from build123d import *

# Parameters (mm, degrees)
SKETCH_1_W          = 120
SKETCH_1_H          = 60
EXTRUDE_1_DEPTH     = 2.5
SKETCH_1_3_W        = 120
SKETCH_1_3_H        = 60
EXTRUDE_2_DEPTH     = 27.5
SKETCH_2_R          = 1.7
CUT_EXTRUDE_1_DEPTH = 74.484692283
SKETCH_3_R          = 1.7
CUT_EXTRUDE_2_DEPTH = 73.5
CUT_EXTRUDE_3_DEPTH = 0.5
SKETCH_5_W          = 2.5
SKETCH_5_H          = 12
CUT_EXTRUDE_4_DEPTH = 8.5
SKETCH_6_R          = 3
CUT_EXTRUDE_5_DEPTH = 15
CHAMFER_1_SIZE      = 2


with BuildPart() as part:
    # 草图1 → 凸台-拉伸1 (new body)
    with BuildSketch(Plane.XY):
        Rectangle(SKETCH_1_W, SKETCH_1_H)
    extrude(amount=-EXTRUDE_1_DEPTH)

    # 草图1<3> → 凸台-拉伸2 (add)
    with BuildSketch(Plane.XY):
        Rectangle(SKETCH_1_3_W, SKETCH_1_3_H)
        with BuildLine():
            Line((-52, 27.5), (52, 27.5))
            Line((52, 27.5), (52, 26))
            ThreePointArc((52, 26), (53.171572875, 23.171572875), (56, 22))
            Line((56, 22), (57.5, 22))
            Line((57.5, 22), (57.5, -22))
            Line((57.5, -22), (56, -22))
            ThreePointArc((56, -22), (53.171572875, -23.171572875), (52, -26))
            Line((52, -26), (52, -27.5))
            Line((52, -27.5), (-52, -27.5))
            Line((-52, -27.5), (-52, -26))
            ThreePointArc((-52, -26), (-53.171572875, -23.171572875), (-56, -22))
            Line((-56, -22), (-57.5, -22))
            Line((-57.5, -22), (-57.5, 22))
            Line((-57.5, 22), (-56, 22))
            ThreePointArc((-56, 22), (-53.171572875, 23.171572875), (-52, 26))
            Line((-52, 26), (-52, 27.5))
        make_face(mode=Mode.SUBTRACT)
    extrude(amount=EXTRUDE_2_DEPTH)

    # 草图2 → 切除-拉伸1 (cut, through all)
    with BuildSketch(Plane.XY.offset(27.5)):
        with Locations((-56, 26)):
            Circle(SKETCH_2_R)
        with Locations((56, 26)):
            Circle(SKETCH_2_R)
        with Locations((56, -26)):
            Circle(SKETCH_2_R)
        with Locations((-56, -26)):
            Circle(SKETCH_2_R)
    extrude(amount=-CUT_EXTRUDE_1_DEPTH, mode=Mode.SUBTRACT)

    # 草图3 → 切除-拉伸2 (cut, through all)
    with BuildSketch(Plane.XY):
        with Locations((-5, 7.5)):
            Circle(SKETCH_3_R)
        with BuildLine():
            Line((52.5, 9.2), (53.5, 9.2))
            ThreePointArc((53.5, 9.2), (55.2, 7.5), (53.5, 5.8))
            Line((53.5, 5.8), (52.5, 5.8))
            ThreePointArc((52.5, 5.8), (50.8, 7.5), (52.5, 9.2))
        make_face()
        with BuildLine():
            Line((52.5, -5.8), (53.5, -5.8))
            ThreePointArc((53.5, -5.8), (55.2, -7.5), (53.5, -9.2))
            Line((53.5, -9.2), (52.5, -9.2))
            ThreePointArc((52.5, -9.2), (50.8, -7.5), (52.5, -5.8))
        make_face()
    extrude(amount=-CUT_EXTRUDE_2_DEPTH, mode=Mode.SUBTRACT)

    # 草图4 → 切除-拉伸3 (cut)
    with BuildSketch(Plane.XY):
        Polygon((-1.8, 7.5), (-3.4, 10.271281292), (-6.6, 10.271281292), (-8.2, 7.5), (-6.6, 4.728718708), (-3.4, 4.728718708), align=None)
        Polygon((56.2, 7.5), (54.6, 10.271281292), (51.4, 10.271281292), (49.8, 7.5), (51.4, 4.728718708), (54.6, 4.728718708), align=None)
        Polygon((56.2, -7.5), (54.6, -4.728718708), (51.4, -4.728718708), (49.8, -7.5), (51.4, -10.271281292), (54.6, -10.271281292), align=None)
    extrude(amount=-CUT_EXTRUDE_3_DEPTH, mode=Mode.SUBTRACT)

    # 草图5 → 切除-拉伸4 (cut)
    with BuildSketch(Plane.XY.offset(27.5)):
        with Locations((58.75, 0)):
            Rectangle(SKETCH_5_W, SKETCH_5_H)
    extrude(amount=-CUT_EXTRUDE_4_DEPTH, mode=Mode.SUBTRACT)

    # 草图6 → 切除-拉伸5 (cut)
    with BuildSketch(Plane(origin=(0, 0, -2.5), x_dir=(-1, 0, 0), z_dir=(0, 0, -1))):
        with Locations((-56, 26)):
            Circle(SKETCH_6_R)
        with Locations((-56, -26)):
            Circle(SKETCH_6_R)
        with Locations((56, -26)):
            Circle(SKETCH_6_R)
        with Locations((56, 26)):
            Circle(SKETCH_6_R)
    extrude(amount=-CUT_EXTRUDE_5_DEPTH, mode=Mode.SUBTRACT)

    # 倒角1
    # the kernel refuses this chamfer: 2 mm, written as the material it takes off along each edge
    with BuildSketch(Plane(origin=(-56, 26, 12.5), x_dir=(1, 0, 0), z_dir=(0, -1, 0))) as chamfer_1_piece_1_section:
        Polygon((1.7, CHAMFER_1_SIZE), (1.7 + CHAMFER_1_SIZE, 0), (1.7, 0), align=None)
    chamfer_1_piece_1 = revolve(axis=Axis((-56, 26, 12.5), (0, 0, 1)), mode=Mode.PRIVATE)
    chamfer_1_piece_1 = chamfer_1_piece_1 & Plane(origin=(-56, 26, 13.857190975), x_dir=(-1, 0, 0), z_dir=(0, 0, -1)) * Cylinder(3, 15, mode=Mode.PRIVATE)
    add(chamfer_1_piece_1, mode=Mode.SUBTRACT)
    with BuildSketch(Plane(origin=(-56, -26, 12.5), x_dir=(1, 0, 0), z_dir=(0, -1, 0))) as chamfer_1_piece_2_section:
        Polygon((1.7, CHAMFER_1_SIZE), (1.7 + CHAMFER_1_SIZE, 0), (1.7, 0), align=None)
    chamfer_1_piece_2 = revolve(axis=Axis((-56, -26, 12.5), (0, 0, 1)), mode=Mode.PRIVATE)
    chamfer_1_piece_2 = chamfer_1_piece_2 & Plane(origin=(-56, -26, 13.857190975), x_dir=(-1, 0, 0), z_dir=(0, 0, -1)) * Cylinder(3, 15, mode=Mode.PRIVATE)
    add(chamfer_1_piece_2, mode=Mode.SUBTRACT)
    with BuildSketch(Plane(origin=(56, -26, 12.5), x_dir=(1, 0, 0), z_dir=(0, -1, 0))) as chamfer_1_piece_3_section:
        Polygon((1.7, CHAMFER_1_SIZE), (1.7 + CHAMFER_1_SIZE, 0), (1.7, 0), align=None)
    chamfer_1_piece_3 = revolve(axis=Axis((56, -26, 12.5), (0, 0, 1)), mode=Mode.PRIVATE)
    chamfer_1_piece_3 = chamfer_1_piece_3 & Plane(origin=(56, -26, 13.857190975), x_dir=(-1, 0, 0), z_dir=(0, 0, -1)) * Cylinder(3, 15, mode=Mode.PRIVATE)
    add(chamfer_1_piece_3, mode=Mode.SUBTRACT)
    with BuildSketch(Plane(origin=(56, 26, 12.5), x_dir=(1, 0, 0), z_dir=(0, -1, 0))) as chamfer_1_piece_4_section:
        Polygon((1.7, CHAMFER_1_SIZE), (1.7 + CHAMFER_1_SIZE, 0), (1.7, 0), align=None)
    chamfer_1_piece_4 = revolve(axis=Axis((56, 26, 12.5), (0, 0, 1)), mode=Mode.PRIVATE)
    chamfer_1_piece_4 = chamfer_1_piece_4 & Plane(origin=(56, 26, 13.857190975), x_dir=(-1, 0, 0), z_dir=(0, 0, -1)) * Cylinder(3, 15, mode=Mode.PRIVATE)
    add(chamfer_1_piece_4, mode=Mode.SUBTRACT)


solid = part.part
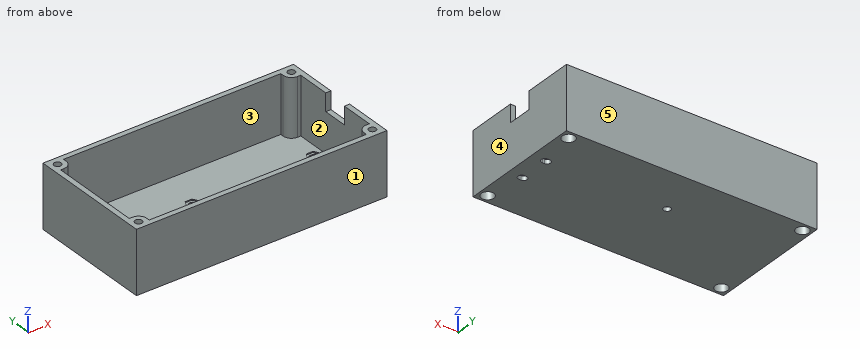
Design review of the part built by this model. Coordinates are the model's own, in mm. Face numbers are marked on the shaded views. A direction names the side the tool comes from. Give positions to 0.01 mm unless a question says otherwise; leave off trailing zeros. Write each loop counter-clockwise with the first axis right and the second up, starting at its lowest first coordinate (ties: lowest second). Pieces come first, ordered by that corner, then holes. Notation, with made-up numbers: M 87.25,20.25 L 129.25,20.25 A20 cw 129.25,45.25 Z; hole C 60.5,72 d10. An arc over 180 degrees is marked long. Answer as a JSON object with one key per item and string values. Group by question number.
1) Clearance check with flat-ended pins moving along their axes: pin 1 Ø3.5 at (x, y) = (56, -26) entering from -Z; pin 2 Ø6 at (x, y) = (-30, -18) entering from +Z. State where each tip first meets the part, or that it passes through.
2) We need section B-B (z = 3). Give the boundary of the cut face in (x, y), and give its area (3 significant figures).
3) We need section C-C (y = -3.5). Give the boundary of the cut face in (x, z), and give its area (3 significant figures).
4) We need section A-A (x = -5). Give the boundary of the cut face in (y, z).
5) We need section D-D (x = -47.5). Give the boundary of the cut face in (y, z).
6) Mouldability with a two-part tool opening along Y and no side actions: class the marked faces 3, 4 and 5 as released by +Y, released by -Y, zero draft, split by the parting line, or undercut.
7) For line 1 along Y through (x, z) = (-56, 20.25); line 2 along X through (y, z) = (26, 8.75); line 3 along Y through (x, z) = (56, 0.75), list the stretches that pass through material, from the lowest coordinate up.
8) Tool access review of the marked faces 1 and 2: name each direction out of +Z, -Z, +X, -X, +Y, -Y from which nothing blocks a thin tool from reaching the whole face with its end or side.
Answer key:
{
 "1": {"pin 1": "stops at z = 14.45", "pin 2": "stops at z = 0"},
 "2": {"outline": "M -60,-30 L 60,-30 L 60,30 L -60,30 Z; hole C -56,-26 d6; hole C -56,26 d6; hole M -57.5,-22 L -56,-22 A4 cw -52,-26 L -52,-27.5 L 52,-27.5 L 52,-26 A4 cw 56,-22 L 57.5,-22 L 57.5,22 L 56,22 A4 cw 52,26 L 52,27.5 L -52,27.5 L -52,26 A4 cw -56,22 L -57.5,22 Z; hole C 56,-26 d6; hole C 56,26 d6", "area": "869 mm²"},
 "3": {"outline": "M -60,-2.5 L 60,-2.5 L 60,19 L 57.5,19 L 57.5,0 L -57.5,0 L -57.5,27.5 L -60,27.5 Z", "area": "416 mm²"},
 "4": {"outline": "M -30,-2.5 L 5.8,-2.5 L 5.8,-0.5 L 4.73,-0.5 L 4.73,0 L -27.5,0 L -27.5,27.5 L -30,27.5 Z; M 9.2,-2.5 L 30,-2.5 L 30,27.5 L 27.5,27.5 L 27.5,0 L 10.27,0 L 10.27,-0.5 L 9.2,-0.5 Z"},
 "5": {"outline": "M -30,-2.5 L 30,-2.5 L 30,27.5 L 27.5,27.5 L 27.5,0 L -27.5,0 L -27.5,27.5 L -30,27.5 Z"},
 "6": {"face 3": "undercut", "face 4": "zero draft", "face 5": "released by +Y"},
 "7": {"line 1": "y = -30 to -27.7, -24.3 to -22, 22 to 24.3, 27.7 to 30", "line 2": "x = -60 to -59, -53 to -52, 52 to 53, 59 to 60", "line 3": "y = -30 to -29, -23 to -22, 22 to 23, 29 to 30"},
 "8": {"face 1": "+Z, -Z, +X, -X, -Y", "face 2": "+Z"}
}
